```python
from build123d import *

# Parameters (mm, degrees)
PIN_CUT_DEPTH                  = 28.640832567
PIN_CUT_DEPTH_BACK             = 28.640832567
SKETCH3_R                      = 1.63195
SKETCH2_R                      = 1.6
F_3MM_CLOSE_FIT_BOLT_CUT_DEPTH = 25.550471012
CHAMFER1_SIZE                  = 0.396875


with BuildPart() as part:
    # Sketch1 → Revolve1 (revolve)
    with BuildSketch(Plane.XY, mode=Mode.PRIVATE) as revolve1_sk:
        Polygon((0, 3.2639), (0, 6.35), (-9.525, 6.35), (-9.525, 16), (-15.875, 16), (-15.875, 5), (-14.0716, 5), (-14.0716, 3.2639), align=None)
    revolve(revolve1_sk.sketch.rotate(Axis((0, 0, 0), (-1, 0, 0)), 90), axis=Axis((0, 0, 0), (-1, 0, 0)))

    # Sketch3 → Pin Cut (cut, two sides: drawn at the far end of the back side and taken through both)
    with BuildSketch(Plane.XY.offset(-PIN_CUT_DEPTH_BACK)):
        with Locations((-4.7625, 0)):
            Circle(SKETCH3_R)
    extrude(amount=PIN_CUT_DEPTH + PIN_CUT_DEPTH_BACK, mode=Mode.SUBTRACT)

    # Sketch2 → 3mm Close Fit Bolt Cut (cut, through all)
    with BuildSketch(Plane(origin=(-9.525, 0, 0), x_dir=(0, 0, -1), z_dir=(1, 0, 0))):
        with Locations((0, 10.082498691)):
            Circle(SKETCH2_R)
        with Locations((-8.7317, -5.041249345)):
            Circle(SKETCH2_R)
        with Locations((8.7317, -5.041249345)):
            Circle(SKETCH2_R)
    extrude(amount=-F_3MM_CLOSE_FIT_BOLT_CUT_DEPTH, mode=Mode.SUBTRACT)

    # Chamfer1
    chamfer1_edges = [part.edges().sort_by_distance(p)[0] for p in [
        (0, 0, 3.2639),
        (-15.875, 0, 16),
        (-9.525, 0, 16),
        (0, 0, 6.35),
    ]]
    chamfer(chamfer1_edges, length=CHAMFER1_SIZE)


solid = part.part
```
Geometry check sheet. Reference: the model listing, model coordinates, mm. A direction names the side the tool comes from. Coordinates: 2 decimals unless noted, no trailing zeros. Order: outer loops, then holes, each group sorted by start corner. A loop starts at its lowest first (then second) coordinate and runs counter-clockwise, first axis right, second up. Notation, with made-up numbers: (71.25, 14) - (82.25, 14) arc R5 cw to (82.25, 23) - close; hole circle Ø5 at (70.25, 64). An arc over 180 degrees is marked (long way). Answer in a Markdown table with one row per item. Add a question column.
1. Access from +Z, -Z, +X, -X, +Y, -Y to the whole of each face (thin tool, end or side, straight path). Record for faces 1 (the face through (-5.025, -1.907, -6.057)), 2 (the face through (-14.072, 1, -3.3)), 3 (the face through (-12.66, -5.65, -10.21)).
2. Section check A-A (z = 0). Give the number of separate pieces and of enclosed holes in the cut face, plus the area to 3 significant figures.
3. Section check C-C (x = -1.5). Enter the section's corners in (y, z).
4. Draft check along Z on faces 4 (the face through (-7.14, -0.14, 3.26)), 5 (the face through (-15.875, -4, 4)), 6 (the face through (-15, 0, 5)), 7 (the face through (-12.74, 15.62, 3.47)). Enter one of: +Z half, -Z half, draft (parallel to the pull), parting line (faces both ways), or undercut.
5. Material ranges on L1, parallel to Z at x = -9.75, y = -5; L2, parallel to X at y = 6.5, z = 0.5 (3 decimals); L3, parallel to X at y = -3.5, z = -2.5, recorded low to high. Write a range as [from, to].
6. Gauge pin test, flat ends, axial feed: pin 1 Ø6 at (y, z) = (-5.5, 5.5) entering from +X; pin 2 Ø4 at (y, z) = (-5.04, 8.73) entering from +X (3 decimals); pin 3 Ø5 at (x, y) = (-4.76, 0) entering from -Z; pin 4 Ø8 at (x, y) = (-2.5, -8.5) entering from -Z. Record the tip position at first contact, or that the pin passes through.
Data:
| question | item | result |
|---|---|---|
| 1 | face 1 | +X |
| 1 | face 2 | -X |
| 1 | face 3 | +X, -X |
| 2 | separate pieces | 3 |
| 2 | enclosed holes | 0 |
| 2 | area | 193 mm² |
| 3 | outline | circle Ø12.7 at (0, 0); hole circle Ø6.53 at (0, 0) |
| 4 | face 4 | undercut |
| 4 | face 5 | draft |
| 4 | face 6 | undercut |
| 4 | face 7 | parting line |
| 5 | L1 | z = [-15.02, -10.33], [-7.13, 7.13], [10.33, 15.02] |
| 5 | L2 | x = [-15.875, -9.525] |
| 5 | L3 | x = [-14.07, 0] |
| 6 | pin 1 | stops at x = 0 |
| 6 | pin 2 | stops at x = -9.525 |
| 6 | pin 3 | stops at z = -6.35 |
| 6 | pin 4 | stops at z = -4.48 |
